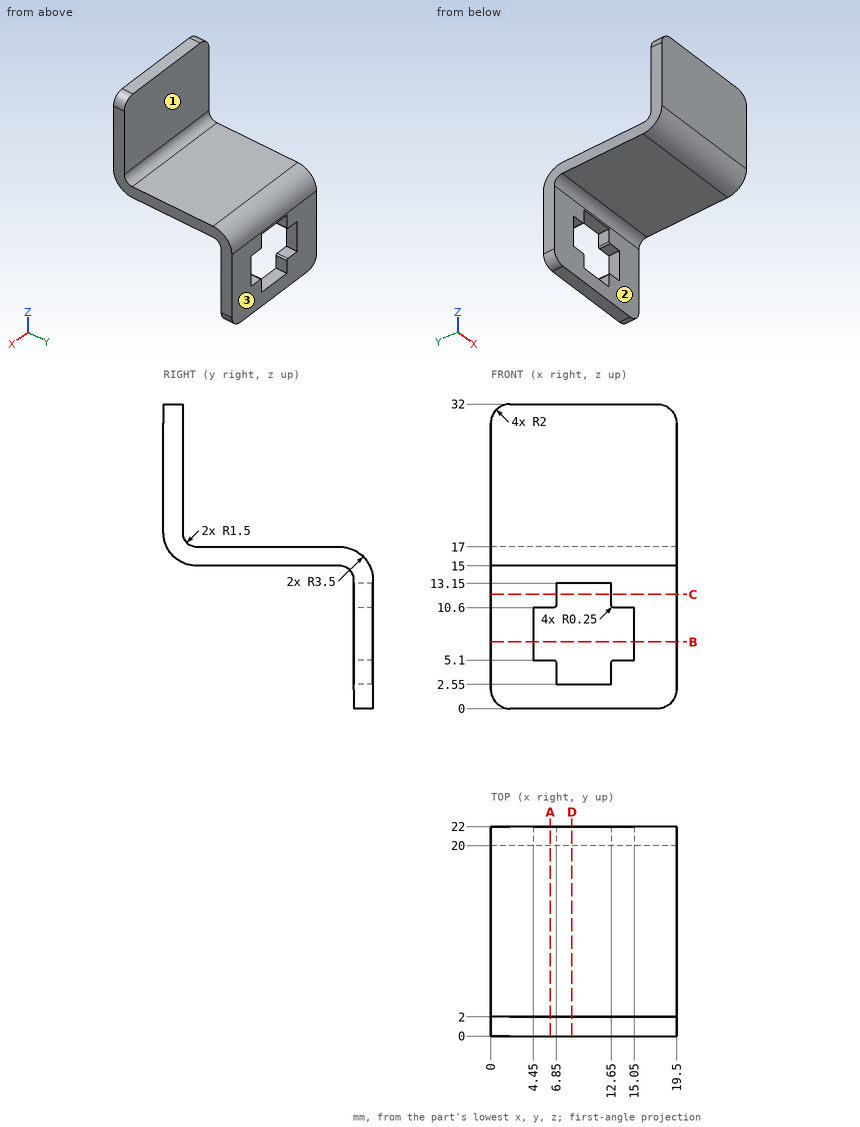
Design review of the part shown in the three views and the two pictorial views. Dimensions are in mm from the part's minimum x, y and z. A direction names the side the tool comes from. Round coordinates to 2 decimals unless told otherwise and drop trailing zeros. Loops run counter-clockwise (first coordinate to the right, second up) from the corner with the lowest first, then second, coordinate; pieces in that order, holes last. Notation, with made-up numbers: M 81,-5.5 L 126,-5.5 A24 cw 126,20.5 Z; hole C 65.5,50.25 d10. An arc over 180 degrees is marked long. Answer as a JSON object with one key per item and string values.
Item 1: We need section A-A on x = 6.25. Give the boundary of the cut face in (y, z).
Answer sheet:
{"outline": "M 0,18.5 A3.5 ccw 3.5,15 L 18.5,15 A1.5 cw 20,13.5 L 20,10.6 L 22,10.6 L 22,13.5 A3.5 ccw 18.5,17 L 3.5,17 A1.5 cw 2,18.5 L 2,32 L 0,32 Z; M 20,0 L 22,0 L 22,5.1 L 20,5.1 Z"}
Item 2: We need section D-D on x = 8.5. Give the boundary of the cut face in (y, z).
Answer sheet:
{"outline": "M 0,18.5 A3.5 ccw 3.5,15 L 18.5,15 A1.5 cw 20,13.5 L 20,13.15 L 22,13.15 L 22,13.5 A3.5 ccw 18.5,17 L 3.5,17 A1.5 cw 2,18.5 L 2,32 L 0,32 Z; M 20,0 L 22,0 L 22,2.55 L 20,2.55 Z"}
Item 3: Wall thickness on L1, parallel to Z at x = 5, y = 10.75; L2, parallel to Y at x = 14.25, z = 22; L3, parallel to Y at x = 8.5, z = 1.5: over which ranges is each line inside the solid? List them lowest first. Write a range as from..to.
Answer sheet:
{"L1": "z = 15..17", "L2": "y = 0..2", "L3": "y = 20..22"}
Item 4: Machinability: for the marked faces 1, 2 and 3, which of the approach directions +Z, -Z, +X, -X, +Y, -Y give a long, thin tool a straight path to every point of the face, cutting with its end or side? Answer none if there is none.
Answer sheet:
{"face 1": "+Z, +X, -X, +Y", "face 2": "-Z, +X, -X, -Y", "face 3": "+Z, -Z, +X, -X, +Y"}
Item 5: We need section B-B on z = 7. Give the boundary of the cut face in (x, y).
Answer sheet:
{"outline": "M 0,20 L 4.45,20 L 4.45,22 L 0,22 Z; M 15.05,20 L 19.5,20 L 19.5,22 L 15.05,22 Z"}
Item 6: Clearance check with flat-ended pins moving along their axes: P1, Ø11, axis at x = 12, z = 24.5, coming from the +Y side; P2, Ø7, axis at x = 5.5, z = 8.5, coming from the -Y side; P3, Ø2, axis at x = 13.5, y = 21, coming from the -Z side; P4, Ø3, axis at x = 10, y = 18, coming from the -Z side. State where each tip first meets the part, or that it passes through.
Answer sheet:
{"P1": "stops at y = 2", "P2": "stops at y = 20", "P3": "stops at z = 0", "P4": "stops at z = 14.62"}
Item 7: We need section C-C on z = 12. Give the boundary of the cut face in (x, y), and give its area (3 significant figures).
Answer sheet:
{"outline": "M 0,20 L 6.85,20 L 6.85,22 L 0,22 Z; M 12.65,20 L 19.5,20 L 19.5,22 L 12.65,22 Z", "area": "27.4 mm^2"}
